```python
from build123d import *

# Parameters (mm, degrees)
F0_W      = 73
F0_H      = 22
F1_DEPTH  = 29
F2_W      = 67
F2_H      = 52
F3_DEPTH  = 19
F4_W      = 58
F4_H      = 4
F5_DEPTH  = 2
F6_W      = 71
F6_H      = 4
F7_DEPTH  = 2
F8_W      = 56
F8_H      = 4
F9_DEPTH  = 2
F10_W     = 69
F10_H     = 4
F11_DEPTH = 2
F12_W     = 42
F12_H     = 28
F13_DEPTH = 22.001
F14_W     = 2.5
F14_H     = 3
F16_W     = 2.5
F16_H     = 3
F18_R     = 1.5
F19_DEPTH = 35.32766
F20_DEPTH = 5.87666
F22_DEPTH = 38.628
F23_W     = 28
F23_H     = 1.5
F24_DEPTH = 2


with BuildPart() as f1:
    # F0 (on Front) → F1 (new body, symmetric)
    with BuildSketch(Plane.XZ):
        Rectangle(F0_W, F0_H)
    extrude(amount=F1_DEPTH, both=True)

    # F2 (on face) → F3 (cut)
    with BuildSketch(Plane.XY.offset(11)):
        Rectangle(F2_W, F2_H)
    extrude(amount=-F3_DEPTH, mode=Mode.SUBTRACT)

    # F4 (on face) → F5 (cut)
    with BuildSketch(Plane.YZ.offset(36.5)):
        with Locations((0, 9)):
            Rectangle(F4_W, F4_H)
    extrude(amount=-F5_DEPTH, mode=Mode.SUBTRACT)

    # F6 (on face) → F7 (cut)
    with BuildSketch(Plane.XZ.offset(29)):
        with Locations((-1, 9)):
            Rectangle(F6_W, F6_H)
    extrude(amount=-F7_DEPTH, mode=Mode.SUBTRACT)

    # F8 (on face) → F9 (cut)
    with BuildSketch(Plane(origin=(-36.5, 0, 0), x_dir=(0, -1, 0), z_dir=(-1, 0, 0))):
        with Locations((-1, 9)):
            Rectangle(F8_W, F8_H)
    extrude(amount=-F9_DEPTH, mode=Mode.SUBTRACT)

    # F10 (on face) → F11 (cut)
    with BuildSketch(Plane(origin=(0, 29, 0), x_dir=(-1, 0, 0), z_dir=(0, 1, 0))):
        with Locations((0, 9)):
            Rectangle(F10_W, F10_H)
    extrude(amount=-F11_DEPTH, mode=Mode.SUBTRACT)

    # F12 (on face) → F13 (cut, through all)
    with BuildSketch(Plane(origin=(0, 0, -11), x_dir=(1, 0, 0), z_dir=(0, 0, -1))):
        with Locations((-12.5, 1)):
            Rectangle(F12_W, F12_H)
    extrude(amount=-F13_DEPTH, mode=Mode.SUBTRACT)

    # F14 (on face) → F15 (revolve)
    with BuildSketch(Plane.XY.offset(-8)):
        with Locations((-32.25, -16.5)):
            Rectangle(F14_W, F14_H)
    revolve(axis=Axis((-31, -16.5, -8), (0, -1, 0)))

    # F16 (on face) → F17 (revolve)
    with BuildSketch(Plane.XY.offset(-8)):
        with Locations((-32.25, 14.5)):
            Rectangle(F16_W, F16_H)
    revolve(axis=Axis((-31, 14.5, -8), (0, 1, 0)))

    # F18 (on face) → F19 (cut)
    with BuildSketch(Plane.XZ.offset(-13)):
        with Locations((-31.0196849202, -7.260261868)):
            Circle(F18_R)
    extrude(amount=F19_DEPTH, mode=Mode.SUBTRACT)

    # F18 (on face) → F20 (cut)
    with BuildSketch(Plane.XZ.offset(-13)):
        with Locations((-31.0196849202, -7.260261868)):
            Circle(F18_R)
    extrude(amount=-F20_DEPTH, mode=Mode.SUBTRACT)

    # F21 (on face) → F22 (cut)
    with BuildSketch(Plane.XZ.offset(18)):
        with BuildLine():
            add(Edge.make_bspline(
                [(-32.3582060158, -6.5832380305), (-32.2676000125, -6.2528454981), (-31.9089266521, -6.0518947977), (-32.1771532814, -5.7944818858)],
                knots=[0, 0, 0, 0, 0.8092690211, 0.8092690211, 0.8092690211, 0.8092690211], degree=3))
            ThreePointArc((-32.3582060158, -6.5832380305), (-31.0196849202, -5.760261868), (-29.6811638245, -6.5832380305))
            add(Edge.make_bspline(
                [(-29.8511186855, -5.7796235172), (-30.1309504135, -6.0518947977), (-29.7859304255, -6.2528454981), (-29.6811638245, -6.5832380305)],
                knots=[0, 0, 0, 0, 0.82138964, 0.82138964, 0.82138964, 0.82138964], degree=3))
            ThreePointArc((-29.8511186855, -5.7796235172), (-31.0159693083, -5.5000510043), (-32.1771532814, -5.7944818858))
        make_face()
    extrude(amount=-F22_DEPTH, mode=Mode.SUBTRACT)

    # F23 (on face) → F24 (join)
    with BuildSketch(Plane(origin=(8.5, 0, 0), x_dir=(0, -1, 0), z_dir=(-1, 0, 0))):
        with Locations((1, -8.75)):
            Rectangle(F23_W, F23_H)
    extrude(amount=F24_DEPTH)


solid = f1.part
```
Here's how the part is built. I have some questions about the finished solid (model axes, mm). A direction names the side the tool comes from. Give positions to 0.01 mm unless a question says otherwise; leave off trailing zeros. Write each loop counter-clockwise with the first axis right and the second up, starting at its lowest first coordinate (ties: lowest second). Pieces come first, ordered by that corner, then holes. Notation, with made-up numbers: M -4.75,19.5 L 0.25,19.5 A27 ccw 0.25,56.5 Z; hole C 48,56 d10. An arc over 180 degrees is marked long. Put each result on its own line as item: value. Start each with the question number.
Item 1: On a 3-axis mill with a long thin cutter (end or side, diameter ignored), from which of +Z, -Z, +X, -X, +Y, -Y can I reach the whole of each face in a straight line? I mean faces 1 (the flat face through (6.5, -1, -9)), 2 (the flat face through (0, -26, 2)), 3 (the flat face through (8, -1, -9.5)). Say none if no direction works.
Item 2: If we section it at B-B, the plane x = -7: Write out the boundary of the cut face in (y, z), then the cut area to 3 significant figures.
Item 3: If we section it at A-A, the plane z = 8.25: Write out the boundary of the cut face in (x, y), then the cut area to 3 significant figures.
Item 4: Will these pins go through, and if not, where does the flat tip stop? pin 1 (1.2 mm diameter, centred on x = -14, z = 10, fed in from +Y); pin 2 (1 mm diameter, centred on y = -22, z = 8, fed in from -X); pin 3 (0.6 mm diameter, centred on x = 7, y = 1.5, fed in from -Z).
Item 5: Thinking about a two-plate mould opening in X: for faces 4 (the flat face through (-34.5, 0, 9)), 5 (the cylindrical face through (-28.874, 14.521, -6.684)), 6 (the flat face through (-1, 29, -2)), which applies, +X half, -X half, draft (parallel to the pull), parting line (faces both ways), or undercut?
Item 6: If we section it at C-C, the plane y = -4: Write out the boundary of the cut face in (x, z).
Item 7: I need wall thicknesses on L1, parallel to Y at x = 2, z = 9.25; L2, parallel to Y at x = 31, z = -7.5; L3, parallel to X at y = -9, z = -7. Which ranges of each line are inside material? Lowest first, please. Write a range as from..to.
Item 8: If we section it at D-D, the plane x = 24: Write out the boundary of the cut face in (y, z), then the cut area to 3 significant figures.
Values:
1. face 1: +Z, -Z
1. face 2: +Z
1. face 3: -Z
2. outline: M -29,-11 L -15,-11 L -15,-8 L -26,-8 L -26,11 L -27,11 L -27,7 L -29,7 Z; M 13,-11 L 29,-11 L 29,7 L 27,7 L 27,11 L 26,11 L 26,-8 L 13,-8 Z
2. area: 188 mm²
3. outline: M -34.5,-27 L 34.5,-27 L 34.5,27 L -34.5,27 Z; hole M -33.5,-26 L 33.5,-26 L 33.5,26 L -33.5,26 Z
3. area: 242 mm²
4. pin 1: y = 27
4. pin 2: x = -34.5
4. pin 3: z = -9.5
5. face 4: -X half
5. face 5: undercut
5. face 6: draft
6. outline: M -36.5,-11 L -33.5,-11 L -33.5,11 L -34.5,11 L -34.5,7 L -36.5,7 Z; M 6.5,-9.5 L 8.5,-9.5 L 8.5,-11 L 36.5,-11 L 36.5,7 L 34.5,7 L 34.5,11 L 33.5,11 L 33.5,-8 L 6.5,-8 Z
7. L1: -27..-26, 26..27
7. L2: -29..-26, 26..29
7. L3: -36.5..-33.5, 33.5..36.5
8. outline: M -29,-11 L 29,-11 L 29,7 L 27,7 L 27,11 L 26,11 L 26,-8 L -26,-8 L -26,11 L -27,11 L -27,7 L -29,7 Z
8. area: 272 mm²
